Geometry: see drawing. Coordinates: mm, zero at the bounding-box minimum. A direction names the side the tool comes from. Give positions to 0.01 mm unless a question says otherwise; leave off trailing zeros. Loops run counter-clockwise (first coordinate to the right, second up) from the corner with the lowest first, then second, coordinate; pieces in that order, holes last. Notation, with made-up numbers: (15.25, 8) -> (64.25, 8) arc R24 cw to (64.25, 23) -> close; hole circle Ø2 at (32.5, -36). An arc over 180 degrees is marked (long way). Return JSON: item names as keys, results as strings. Group by question number.
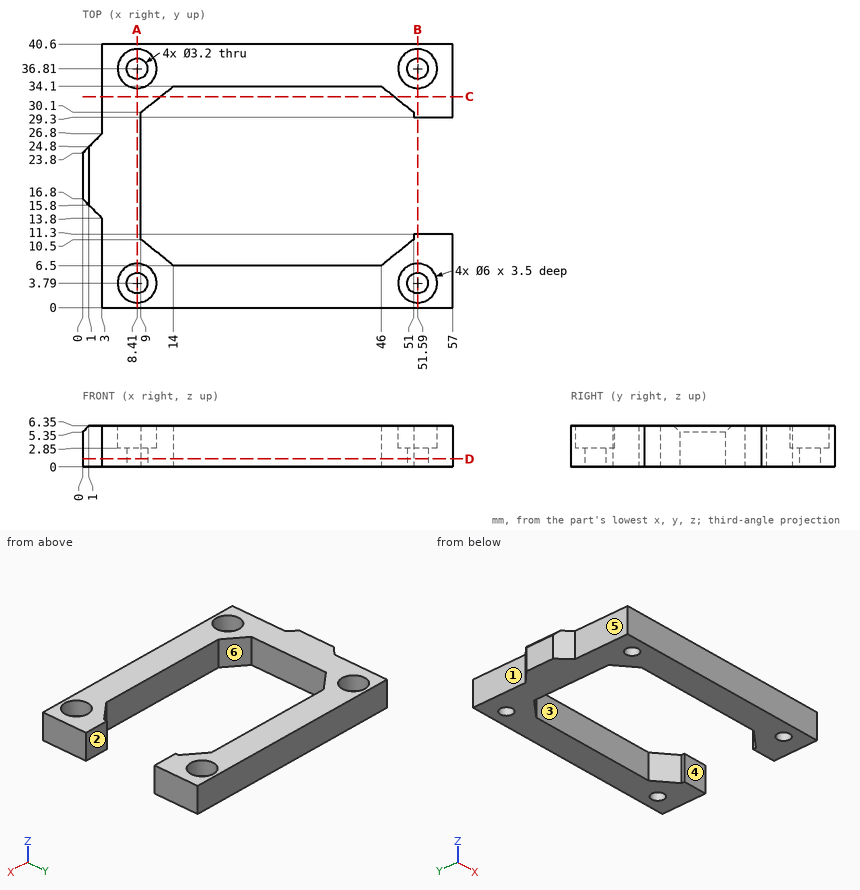
1) Cut plane D-D on z = 1.25. Return loops of the section in (x, y).
2) Mould query, pull axis X, two halves, no side actions, for the marked faces 4, 5 and 6. Classes: released by +X, released by -X, zero draft, split by the parting line, or undercut.
3) Material intervals for line 1 (Y direction, x = 8.41, z = 1.6); line 2 (Y direction, x = 51.59, z = 1.45); line 3 (Y direction, x = 21, z = 0.5), sorted ascending.
4) Cut plane A-A on x = 8.41. Return loops of the section in (y, z).
5) Cut plane B-B on x = 51.59. Return loops of the section in (y, z), then the cut area to 3 significant figures.
6) Contact query for flat-ended pins moving along their axis: P1, Ø3, axis at y = 34, z = 4.5, coming from the -X side; P2, Ø4, axis at x = 8.41, y = 3.79, coming from the +Z side. Output: stop coordinate, or through.
7) Reachability of the marked faces 1, 2 and 3 from +Z, -Z, +X, -X, +Y, -Y: full face, straight path, thin tool, end or side. Return the list, or none.
8) Cut plane C-C on y = 32.5. Return loops of the section in (x, z), then the cut area to 3 significant figures.
Calculated:
{
 "1": {"outline": "(0, 16.8) -> (3, 13.8) -> (3, 0) -> (57, 0) -> (57, 11.3) -> (51, 11.3) -> (51, 10.5) -> (46, 6.5) -> (14, 6.5) -> (9, 10.5) -> (9, 30.1) -> (14, 34.1) -> (46, 34.1) -> (51, 30.1) -> (51, 29.3) -> (57, 29.3) -> (57, 40.6) -> (3, 40.6) -> (3, 26.8) -> (0, 23.8) -> close; hole circle Ø3.2 at (8.41, 3.79); hole circle Ø3.2 at (8.41, 36.81); hole circle Ø3.2 at (51.59, 3.79); hole circle Ø3.2 at (51.59, 36.81)"},
 "2": {"face 4": "zero draft", "face 5": "released by -X", "face 6": "undercut"},
 "3": {"line 1": "0 to 2.19, 5.39 to 35.21, 38.41 to 40.6", "line 2": "0 to 2.19, 5.39 to 11.3, 29.3 to 35.21, 38.41 to 40.6", "line 3": "0 to 6.5, 34.1 to 40.6"},
 "4": {"outline": "(0, 0) -> (2.19, 0) -> (2.19, 2.85) -> (0.79, 2.85) -> (0.79, 6.35) -> (0, 6.35) -> close; (5.39, 0) -> (35.21, 0) -> (35.21, 2.85) -> (33.81, 2.85) -> (33.81, 6.35) -> (6.79, 6.35) -> (6.79, 2.85) -> (5.39, 2.85) -> close; (38.41, 0) -> (40.6, 0) -> (40.6, 6.35) -> (39.81, 6.35) -> (39.81, 2.85) -> (38.41, 2.85) -> close"},
 "5": {"outline": "(0, 0) -> (2.19, 0) -> (2.19, 2.85) -> (0.79, 2.85) -> (0.79, 6.35) -> (0, 6.35) -> close; (5.39, 0) -> (11.3, 0) -> (11.3, 6.35) -> (6.79, 6.35) -> (6.79, 2.85) -> (5.39, 2.85) -> close; (29.3, 0) -> (35.21, 0) -> (35.21, 2.85) -> (33.81, 2.85) -> (33.81, 6.35) -> (29.3, 6.35) -> close; (38.41, 0) -> (40.6, 0) -> (40.6, 6.35) -> (39.81, 6.35) -> (39.81, 2.85) -> (38.41, 2.85) -> close", "area": "83.3 mm2"},
 "6": {"P1": "x = 3", "P2": "z = 2.85"},
 "7": {"face 1": "+Z, -Z, -X, +Y", "face 2": "+Z, -Z, +X", "face 3": "+Z, -Z"},
 "8": {"outline": "(3, 0) -> (12, 0) -> (12, 6.35) -> (3, 6.35) -> close; (48, 0) -> (57, 0) -> (57, 6.35) -> (48, 6.35) -> close", "area": "114 mm2"}
}
